Can you work these out from the model? Positions are in its coordinate system, mm. A direction names the side the tool comes from. Round coordinates to 2 decimals unless told otherwise and drop trailing zeros. Order: outer loops, then holes, each group sorted by start corner. A loop starts at its lowest first (then second) coordinate and runs counter-clockwise, first axis right, second up. Notation, with made-up numbers: (55, 77.25) - (72, 77.25) arc R23 cw to (72, 107.25) - close; hole circle Ø3 at (-19.75, 39). An arc over 180 degrees is marked (long way). Write item = value, one per line.
from build123d import *

# Parameters (mm, degrees)
F0_R     = 1.050001
F1_DEPTH = 2
F0_W     = 85
F0_H     = 45
F2_DEPTH = 3


with BuildPart() as f1:
    # F0 (on Top) → F1 (new body)
    with BuildSketch(Plane.XY):
        with BuildLine():
            ThreePointArc((55, 32), (54.12132, 34.12132), (52, 35))
            Line((52, 35), (-52, 35))
            ThreePointArc((-52, 35), (-54.12132, 34.12132), (-55, 32))
            Line((-55, 32), (-55, -32))
            ThreePointArc((-55, -32), (-54.12132, -34.12132), (-52, -35))
            Line((-52, -35), (52, -35))
            ThreePointArc((52, -35), (54.12132, -34.12132), (55, -32))
            Line((55, -32), (55, 32))
        make_face()
        with Locations((-51.286835, -31.298466)):
            Circle(F0_R, mode=Mode.SUBTRACT)
        with Locations((51.286835, -31.298466)):
            Circle(F0_R, mode=Mode.SUBTRACT)
        with Locations((-51.286835, 31.298466)):
            Circle(F0_R, mode=Mode.SUBTRACT)
        with BuildLine():
            ThreePointArc((47.451668, 32.600001), (48.427401, 28.430343), (52.600001, 27.467266))
            Line((52.600001, 27.467266), (52.600001, -27.467266))
            ThreePointArc((52.600001, -27.467266), (48.427401, -28.430343), (47.451668, -32.600001))
            Line((47.451668, -32.600001), (-47.451668, -32.600001))
            ThreePointArc((-47.451668, -32.600001), (-48.427401, -28.430343), (-52.600001, -27.467266))
            Line((-52.600001, -27.467266), (-52.600001, 27.467266))
            ThreePointArc((-52.600001, 27.467266), (-48.427401, 28.430343), (-47.451668, 32.600001))
            Line((-47.451668, 32.600001), (47.451668, 32.600001))
        make_face(mode=Mode.SUBTRACT)
        with Locations((51.286835, 31.298466)):
            Circle(F0_R, mode=Mode.SUBTRACT)
    extrude(amount=F1_DEPTH)

    # F0 (on Top) → F2 (join)
    with BuildSketch(Plane.XY):
        with BuildLine():
            Line((52.600001, -27.467266), (52.600001, 27.467266))
            ThreePointArc((52.600001, 27.467266), (48.427401, 28.430343), (47.451668, 32.600001))
            Line((47.451668, 32.600001), (-47.451668, 32.600001))
            ThreePointArc((-47.451668, 32.600001), (-48.427401, 28.430343), (-52.600001, 27.467266))
            Line((-52.600001, 27.467266), (-52.600001, -27.467266))
            ThreePointArc((-52.600001, -27.467266), (-48.427401, -28.430343), (-47.451668, -32.600001))
            Line((-47.451668, -32.600001), (47.451668, -32.600001))
            ThreePointArc((47.451668, -32.600001), (48.427401, -28.430343), (52.600001, -27.467266))
        make_face()
        Rectangle(F0_W, F0_H, mode=Mode.SUBTRACT)
    extrude(amount=F2_DEPTH)


solid = f1.part
(1) If we section it at A-A (y = -2.5): Write out the boundary of the cut face in (x, z), plus the area to 3 significant figures.
Computed:
outline = (-55, 0) - (-42.5, 0) - (-42.5, 3) - (-52.6, 3) - (-52.6, 2) - (-55, 2) - close; (42.5, 0) - (55, 0) - (55, 2) - (52.6, 2) - (52.6, 3) - (42.5, 3) - close
area = 70.2 mm^2
(2) If I drill on line 1 (Y direction, x = -14.5, z = 1); line 2 (X direction, y = -18.5, z = 1.6); line 3 (Y direction, x = -18, z = 2.3), over which ranges is the centre line in solid material (lowest first)? Write a range as from..to.
Computed:
line_1 = -35..-22.5, 22.5..35
line_2 = -55..-42.5, 42.5..55
line_3 = -32.6..-22.5, 22.5..32.6
(3) If we section it at C-C (z = 1.1): Write out the boundary of the cut face in (x, y).
Computed:
outline = (-55, -32) arc R3 ccw to (-52, -35) - (52, -35) arc R3 ccw to (55, -32) - (55, 32) arc R3 ccw to (52, 35) - (-52, 35) arc R3 ccw to (-55, 32) - close; hole circle Ø2.1 at (-51.29, -31.3); hole circle Ø2.1 at (-51.29, 31.3); hole (-42.5, -22.5) - (42.5, -22.5) - (42.5, 22.5) - (-42.5, 22.5) - close; hole circle Ø2.1 at (51.29, -31.3); hole circle Ø2.1 at (51.29, 31.3)
(4) Thinking about a two-plate mould opening in X: for faces 4 (the face through (-54.1, 34.14, 0.99)), 5 (the face through (50.513, 32.008, 0.986)), 6 (the face through (54.14, 34.1, 0.99)), which applies, +X half, -X half, draft (parallel to the pull), parting line (faces both ways), or undercut?
Computed:
face_4 = -X half
face_5 = undercut
face_6 = +X half
(5) Will these pins go through, and if not, where does the flat tip stop? P1, Ø1.9, axis at x = -51.29, y = 31.3, coming from the +Z side; P2, Ø0.5, axis at x = -17, z = 2.5, coming from the +Y side; P3, Ø2.5, axis at x = 51.29, y = 31.3, coming from the +Z side.
Computed:
P1 = through
P2 = 32.6
P3 = 2
(6) On a 3-axis mill with a long thin cutter (end or side, diameter ignored), from which of +Z, -Z, +X, -X, +Y, -Y can I reach the whole of each face in a straight line? I mean faces 1 (the face through (-48.47, -28.39, 2.49)), 2 (the face through (-42.5, 0, 1)), 3 (the face through (54.1, -34.14, 0.99)). Say none if no direction works.
Computed:
face_1 = +Z
face_2 = +Z, -Z
face_3 = +Z, -Z, +X, -Y
(7) If we section it at B-B (x = 20.5): Write out the boundary of the cut face in (y, z), plus the area to 3 significant figures.
Computed:
outline = (-35, 0) - (-22.5, 0) - (-22.5, 3) - (-32.6, 3) - (-32.6, 2) - (-35, 2) - close; (22.5, 0) - (35, 0) - (35, 2) - (32.6, 2) - (32.6, 3) - (22.5, 3) - close
area = 70.2 mm^2
